The model under review builds one solid part; all positions refer to its coordinate system, in mm. Coordinates: 2 decimals unless noted, no trailing zeros. Order: outer loops, then holes, each group sorted by start corner. A loop starts at its lowest first (then second) coordinate and runs counter-clockwise, first axis right, second up. Notation, with made-up numbers: (-17, -38.5) - (35, -38.5) arc R12 ccw to (35, -32.5) - close; hole circle Ø9 at (0.25, -23.5). An arc over 180 degrees is marked (long way). Answer in a Markdown table with one row per item.
```python
from build123d import *

# Parameters (mm, degrees)
SKETCH1_W           = 70
SKETCH1_H           = 70
BOSS_EXTRUDE1_DEPTH = 0.08
SKETCH2_R           = 3
CUT_EXTRUDE1_DEPTH  = 10
FILLET1_R           = 3
SKETCH3_R           = 4
CUT_EXTRUDE2_DEPTH  = 10


with BuildPart() as part:
    # Sketch1 → Boss-Extrude1 (new body)
    with BuildSketch(Plane.XY):
        Rectangle(SKETCH1_W, SKETCH1_H)
    extrude(amount=BOSS_EXTRUDE1_DEPTH)

    # Sketch2 → Cut-Extrude1 (cut)
    with BuildSketch(Plane.XY.offset(0.08)):
        with Locations((0, 25)):
            Circle(SKETCH2_R)
        with Locations((25, 25)):
            Circle(SKETCH2_R)
        with Locations((25, 0)):
            Circle(SKETCH2_R)
        with Locations((-25, 0)):
            Circle(SKETCH2_R)
        with Locations((-25, 25)):
            Circle(SKETCH2_R)
        with Locations((-25, -25)):
            Circle(SKETCH2_R)
        with Locations((0, -25)):
            Circle(SKETCH2_R)
        with Locations((25, -25)):
            Circle(SKETCH2_R)
    extrude(amount=-CUT_EXTRUDE1_DEPTH, mode=Mode.SUBTRACT)

    # Fillet1
    fillet1_edges = [part.edges().sort_by_distance(p)[0] for p in [
        (35, -35, 0.04),
        (-35, -35, 0.04),
        (-35, 35, 0.04),
        (35, 35, 0.04),
    ]]
    fillet(fillet1_edges, radius=FILLET1_R)

    # Sketch3 → Cut-Extrude2 (cut)
    with BuildSketch(Plane(origin=(0, 0, 0), x_dir=(-1, 0, 0), z_dir=(0, 0, -1))):
        with Locations((20, 10)):
            Circle(SKETCH3_R)
        with Locations((-20, -10)):
            Circle(SKETCH3_R)
    extrude(amount=-CUT_EXTRUDE2_DEPTH, mode=Mode.SUBTRACT)


solid = part.part
```
Item 1: Clearance check with a flat-ended pin moving along its axis: pin 1 Ø9.5 at (x, y) = (25, 0) entering from +Z. State where the tip first meets the part, or that it passes through.
Check values:
| item | result |
|---|---|
| pin 1 | z = 0.08 |
Item 2: We need section A-A, the plane x = 25. Write out the cut boundary in (y, z).
Check values:
| item | result |
|---|---|
| outline | (-35, 0) - (-28, 0) - (-28, 0.08) - (-35, 0.08) - close; (-22, 0) - (-3, 0) - (-3, 0.08) - (-22, 0.08) - close; (3, 0) - (22, 0) - (22, 0.08) - (3, 0.08) - close; (28, 0) - (35, 0) - (35, 0.08) - (28, 0.08) - close |
Item 3: We need section C-C, the plane x = 0. Write out the cut boundary in (y, z).
Check values:
| item | result |
|---|---|
| outline | (-35, 0) - (-28, 0) - (-28, 0.08) - (-35, 0.08) - close; (-22, 0) - (22, 0) - (22, 0.08) - (-22, 0.08) - close; (28, 0) - (35, 0) - (35, 0.08) - (28, 0.08) - close |
Item 4: We need section D-D, the plane y = 10. Write out the cut boundary in (x, z), then the cut area to 3 significant figures.
Check values:
| item | result |
|---|---|
| outline | (-35, 0) - (-24, 0) - (-24, 0.08) - (-35, 0.08) - close; (-16, 0) - (35, 0) - (35, 0.08) - (-16, 0.08) - close |
| area | 4.96 mm^2 |
